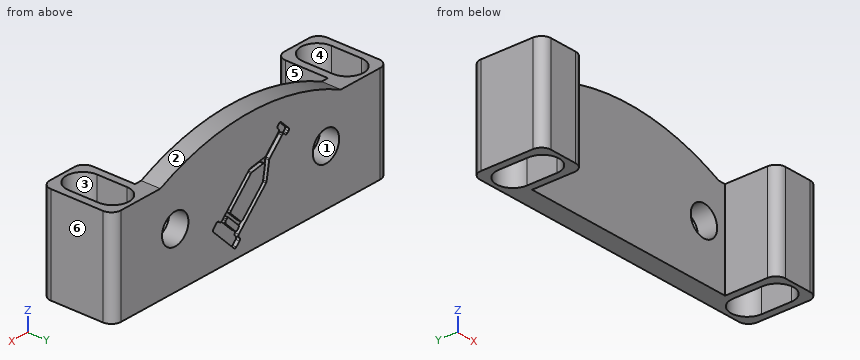
```python
from build123d import *

# Parameters (mm, degrees)
SKETCH_1_W          = 27.112781954
SKETCH_1_H          = 9.518796992
SKETCH_1_R          = 1.575
EXTRUDE_1_DEPTH     = 2
SKETCH_2_W          = 27.112781954
SKETCH_2_H          = 2
EXTRUDE_2_DEPTH     = 0.91
CUT_EXTRUDE_1_DEPTH = 15.829626281
CUT_EXTRUDE_2_DEPTH = 17.785702449
EXTRUDE_3_DEPTH     = 10
SKETCH_8_R          = 1.575
CUT_EXTRUDE_3_DEPTH = 10
EXTRUDE_4_DEPTH     = 2
FILLET_2_R          = 1
CUT_EXTRUDE_4_DEPTH = 0.4


with BuildPart() as part:
    # Эскиз1 → Бобышка-Вытянуть1 (new body)
    with BuildSketch(Plane(origin=(0, 0, 0), x_dir=(1, 0, 0), z_dir=(0, 1, 0))):
        Rectangle(SKETCH_1_W, SKETCH_1_H)
        with Locations(Location((-9, 0, 0), (0, 0, 270))):
            Circle(SKETCH_1_R, mode=Mode.SUBTRACT)
        with Locations(Location((9, 0, 0), (0, 0, 270))):
            Circle(SKETCH_1_R, mode=Mode.SUBTRACT)
    extrude(amount=EXTRUDE_1_DEPTH)

    # Эскиз2 → Бобышка-Вытянуть2 (add)
    with BuildSketch(Plane(origin=(0, 0, -4.759398496), x_dir=(-1, 0, 0), z_dir=(0, 0, -1))):
        with Locations((0, 1)):
            Rectangle(SKETCH_2_W, SKETCH_2_H)
    extrude(amount=EXTRUDE_2_DEPTH)

    # Эскиз3 → Вырез-Вытянуть1 (cut, through all)
    with BuildSketch(Plane.XZ):
        Polygon((-6.720997268, 4.759398496), (-3, 5.765), (-14.556442119, 5.765), (-14.556442119, -5.765), (-3, -5.765), (-3.353751395, -5.669398496), (-13.556390977, -5.669398496), (-13.556390977, 4.759398496), align=None)
        with BuildLine():
            Line((-10.043565082, 3.861472766), (-6.720997268, 4.759398496))
            Line((-6.720997268, 4.759398496), (-13.556390977, 4.759398496))
            Line((-13.556390977, 4.759398496), (-13.556390977, -5.669398496))
            Line((-13.556390977, -5.669398496), (-3.353751395, -5.669398496))
            Line((-3.353751395, -5.669398496), (-10.043565082, -3.861472766))
            ThreePointArc((-10.043565082, -3.861472766), (-13, 0), (-10.043565082, 3.861472766))
        make_face()
        with BuildLine():
            Line((13.556390977, 4.759398496), (6.720997268, 4.759398496))
            Line((6.720997268, 4.759398496), (10.043565082, 3.861472766))
            ThreePointArc((10.043565082, 3.861472766), (12.17602427, 2.431639331), (13, 0))
            ThreePointArc((13, 0), (12.17602427, -2.431639331), (10.043565082, -3.861472766))
            Line((10.043565082, -3.861472766), (3.353751395, -5.669398496))
            Line((3.353751395, -5.669398496), (13.556390977, -5.669398496))
            Line((13.556390977, -5.669398496), (13.556390977, 4.759398496))
        make_face()
        Polygon((3, 5.765), (6.720997268, 4.759398496), (13.556390977, 4.759398496), (13.556390977, -5.669398496), (3.353751395, -5.669398496), (3, -5.765), (14.556442119, -5.765), (14.556442119, 5.765), align=None)
    extrude(amount=-CUT_EXTRUDE_1_DEPTH, mode=Mode.SUBTRACT)

    # Эскиз4 → Вырез-Вытянуть2 (cut, through all)
    with BuildSketch(Plane(origin=(0, 0, -5.669398496), x_dir=(-1, 0, 0), z_dir=(0, 0, -1))):
        Polygon((11.521782541, 2), (11.521782541, -6.403006286), (13.618299284, -6.403006286), (13.618299284, 3.686124148), (11.521782541, 3.686124148), align=None)
        Polygon((-13.618299284, -6.403006286), (-11.521782541, -6.403006286), (-11.521782541, 2), (-11.521782541, 3.686124148), (-13.618299284, 3.686124148), align=None)
    extrude(amount=-CUT_EXTRUDE_2_DEPTH, mode=Mode.SUBTRACT)

    # Эскиз7 → Бобышка-Вытянуть3 (add)
    with BuildSketch(Plane(origin=(0, 0, -5.669398496), x_dir=(-1, 0, 0), z_dir=(0, 0, -1))):
        Polygon((3.353751395, 0), (11.521782541, 0), (11.521782541, -5.430586026), (16.478217459, -5.430586026), (16.478217459, 2), (11.521782541, 2), (3.353751395, 2), align=None)
        with BuildLine():
            Line((15.7, -3.265293013), (15.7, -0.165293013))
            ThreePointArc((15.7, -0.165293013), (14, 1.534706987), (12.3, -0.165293013))
            Line((12.3, -0.165293013), (12.3, -3.265293013))
            ThreePointArc((12.3, -3.265293013), (14, -4.965293013), (15.7, -3.265293013))
        make_face(mode=Mode.SUBTRACT)
    extrude_3 = extrude(amount=-EXTRUDE_3_DEPTH)

    # Эскиз8 → Вырез-Вытянуть3 (cut)
    with BuildSketch(Plane(origin=(0, 2, 0), x_dir=(1, 0, 0), z_dir=(0, 1, 0))):
        with Locations(Location((-9, 0, 0), (0, 0, 270))):
            Circle(SKETCH_8_R)
    cut_extrude_3 = extrude(amount=-CUT_EXTRUDE_3_DEPTH, mode=Mode.SUBTRACT)

    # Зеркальное отражение1: Бобышка-Вытянуть3, Вырез-Вытянуть3 across plane
    add(extrude_3.mirror(Plane(origin=(0, 0, 0), x_dir=(0, 0, 1), z_dir=(1, 0, 0))))
    add(cut_extrude_3.mirror(Plane(origin=(0, 0, 0), x_dir=(0, 0, 1), z_dir=(1, 0, 0))), mode=Mode.SUBTRACT)

    # Эскиз9 → Бобышка-Вытянуть4 (add)
    with BuildSketch(Plane(origin=(0, 2, 0), x_dir=(1, 0, 0), z_dir=(0, 1, 0))):
        with BuildLine():
            Line((6.720997268, -4.759398496), (-6.720997268, -4.759398496))
            Line((-6.720997268, -4.759398496), (-8.307661997, -4.330601504))
            Line((-8.307661997, -4.330601504), (-10.777839616, -4.330601504))
            ThreePointArc((-10.777839616, -4.330601504), (0, -6.773159867), (10.777839616, -4.330601504))
            Line((10.777839616, -4.330601504), (8.307661997, -4.330601504))
            Line((8.307661997, -4.330601504), (6.720997268, -4.759398496))
        make_face()
    extrude(amount=-EXTRUDE_4_DEPTH)

    # Скругление2
    fillet_2_edges = [part.edges().sort_by_distance(p)[0] for p in [
        (-16.478217459, 2, -0.669398496),
        (-16.478217459, -5.430586026, -0.669398496),
        (-11.521782541, -5.430586026, -0.669398496),
        (11.521782541, -5.430586026, -0.669398496),
        (16.478217459, -5.430586026, -0.669398496),
        (16.478217459, 2, -0.669398496),
    ]]
    fillet(fillet_2_edges, radius=FILLET_2_R)

    # Эскиз12 → Вырез-Вытянуть4 (cut)
    with BuildSketch(Plane(origin=(0, 2, 0), x_dir=(1, 0, 0), z_dir=(0, 1, 0))):
        with BuildLine():
            Line((4.446560813, 2.176089775), (1.988755362, 4.633895225))
            ThreePointArc((1.988755362, 4.633895225), (1.847334006, 4.692473869), (1.70591265, 4.633895225))
            Line((1.70591265, 4.633895225), (1.327376273, 4.255358849))
            ThreePointArc((1.327376273, 4.255358849), (1.268797629, 4.113937492), (1.327376273, 3.972516136))
            Line((1.327376273, 3.972516136), (1.402795262, 3.897097148))
            ThreePointArc((1.402795262, 3.897097148), (1.461373905, 3.755675791), (1.402795262, 3.614254435))
            Line((1.402795262, 3.614254435), (-1.852293326, 0.359165847))
            ThreePointArc((-1.852293326, 0.359165847), (-1.888439649, 0.309775569), (-1.907956953, 0.25176668))
            Line((-1.907956953, 0.25176668), (-2.218358166, -1.546336835))
            ThreePointArc((-2.218358166, -1.546336835), (-2.23787547, -1.604345724), (-2.274021793, -1.653736003))
            Line((-2.274021793, -1.653736003), (-3.75824321, -3.13795742))
            ThreePointArc((-3.75824321, -3.13795742), (-3.899664566, -3.196536063), (-4.041085922, -3.13795742))
            Line((-4.041085922, -3.13795742), (-4.109500023, -3.069543319))
            ThreePointArc((-4.109500023, -3.069543319), (-4.250921379, -3.010964675), (-4.392342735, -3.069543319))
            Line((-4.392342735, -3.069543319), (-4.522380617, -3.1995812))
            ThreePointArc((-4.522380617, -3.1995812), (-4.58095926, -3.341002556), (-4.522380617, -3.482423913))
            Line((-4.522380617, -3.482423913), (-3.669758325, -4.335046204))
            ThreePointArc((-3.669758325, -4.335046204), (-3.528336969, -4.393624848), (-3.386915613, -4.335046204))
            Line((-3.386915613, -4.335046204), (-3.256877732, -4.205008323))
            ThreePointArc((-3.256877732, -4.205008323), (-3.198299088, -4.063586966), (-3.256877732, -3.92216561))
            Line((-3.256877732, -3.92216561), (-3.325291832, -3.853751509))
            ThreePointArc((-3.325291832, -3.853751509), (-3.383870476, -3.712330153), (-3.325291832, -3.570908797))
            Line((-3.325291832, -3.570908797), (-1.841070415, -2.08668738))
            ThreePointArc((-1.841070415, -2.08668738), (-1.791680137, -2.050541057), (-1.733671248, -2.031023753))
            Line((-1.733671248, -2.031023753), (0.064432267, -1.720622541))
            ThreePointArc((0.064432267, -1.720622541), (0.122441156, -1.701105237), (0.171831435, -1.664958913))
            Line((0.171831435, -1.664958913), (3.426920022, 1.590129674))
            ThreePointArc((3.426920022, 1.590129674), (3.568341379, 1.648708318), (3.709762735, 1.590129674))
            Line((3.709762735, 1.590129674), (3.785181724, 1.514710686))
            ThreePointArc((3.785181724, 1.514710686), (3.92660308, 1.456132042), (4.068024436, 1.514710686))
            Line((4.068024436, 1.514710686), (4.446560813, 1.893247062))
            ThreePointArc((4.446560813, 1.893247062), (4.505139456, 2.034668419), (4.446560813, 2.176089775))
        make_face()
        with BuildLine():
            Line((2.963799211, 2.036003209), (1.848668796, 3.151133624))
            ThreePointArc((1.848668796, 3.151133624), (1.70724744, 3.209712267), (1.565826084, 3.151133624))
            Line((1.565826084, 3.151133624), (1.465360653, 3.050668193))
            ThreePointArc((1.465360653, 3.050668193), (1.406782009, 2.909246836), (1.465360653, 2.76782548))
            Line((1.465360653, 2.76782548), (2.580491067, 1.652695065))
            ThreePointArc((2.580491067, 1.652695065), (2.721912424, 1.594116422), (2.86333378, 1.652695065))
            Line((2.86333378, 1.652695065), (2.963799211, 1.753160497))
            ThreePointArc((2.963799211, 1.753160497), (3.022377855, 1.894581853), (2.963799211, 2.036003209))
        make_face(mode=Mode.SUBTRACT)
        with BuildLine():
            Line((2.334078689, 1.406282687), (1.218948275, 2.521413102))
            ThreePointArc((1.218948275, 2.521413102), (1.077526918, 2.579991746), (0.936105562, 2.521413102))
            Line((0.936105562, 2.521413102), (-1.42428076, 0.16102678))
            ThreePointArc((-1.42428076, 0.16102678), (-1.460427083, 0.111636501), (-1.479944387, 0.053627613))
            Line((-1.479944387, 0.053627613), (-1.712610446, -1.294168861))
            ThreePointArc((-1.712610446, -1.294168861), (-1.656946819, -1.469612406), (-1.481503274, -1.525276034))
            Line((-1.481503274, -1.525276034), (-0.1337068, -1.292609974))
            ThreePointArc((-0.1337068, -1.292609974), (-0.075697911, -1.27309267), (-0.026307633, -1.236946347))
            Line((-0.026307633, -1.236946347), (2.334078689, 1.123439975))
            ThreePointArc((2.334078689, 1.123439975), (2.392657333, 1.264861331), (2.334078689, 1.406282687))
        make_face(mode=Mode.SUBTRACT)
    extrude(amount=-CUT_EXTRUDE_4_DEPTH, mode=Mode.SUBTRACT)


solid = part.part
```
The listing builds one solid part. Answer for the finished solid, in the listing's coordinates (mm). Face numbers are marked on the shaded views. A direction names the side the tool comes from. Give positions to 0.01 mm unless a question says otherwise; leave off trailing zeros. Write each loop counter-clockwise with the first axis right and the second up, starting at its lowest first coordinate (ties: lowest second). Pieces come first, ordered by that corner, then holes. Notation, with made-up numbers: M 23,-17.75 L 53,-17.75 A31 cw 53,9.25 Z; hole C -23.5,33.25 d11. An arc over 180 degrees is marked long. Write each question's results on one line, items separated by ' | '.
Q1. Section A-A, the plane x = -14 is taken. Write down the section's boundary in (y, z).
Output values:
outline: M -5.43,-5.67 L -4.97,-5.67 L -4.97,4.33 L -5.43,4.33 Z; M 1.53,-5.67 L 2,-5.67 L 2,4.33 L 1.53,4.33 Z
Q2. Flat-ended cylindrical pins translate along their axes: P1, Ø3, axis at x = -5.5, z = -3, coming from the -Y side; P2, Ø3, axis at x = 9, z = 0, coming from the -Y side. Find the tip coordinate at first contact, or state that the pin passes through.
Output values:
P1: y = 0 | P2: through
Q3. A tool of negligible diameter and unlimited length cuts with its end or side. For the marked faces 4, 5 and 6, from which of +Z, -Z, +X, -X, +Y, -Y can it reach the whole face along a straight path? Write none if from no direction.
Output values:
face 4: +Z, -Z | face 5: +Z, -Z, -Y | face 6: +Z, -Z, +X, +Y, -Y
Q4. Consider L1, parallel to X at y = -1.5, z = 0.5; L2, parallel to X at y = -4.25, z = 2.5; L3, parallel to Y at x = 14, z = 4.25. Determine where each line is inside the solid, lowest interval first. Write a range as from..to.
Output values:
L1: -16.48..-15.7, -12.3..-11.52, 11.52..12.3, 15.7..16.48 | L2: -16.48..-15.39, -12.61..-11.52, 11.52..12.61, 15.39..16.48 | L3: -5.43..-4.97, 1.53..2
Q5. Section C-C, the plane x = 9 is taken. Write down the section's boundary in (y, z) (3 decimals).
Output values:
outline: M 0,-5.669 L 2,-5.669 L 2,-1.575 L 0,-1.575 Z; M 0,1.575 L 2,1.575 L 2,5.097 L 0,5.097 Z
Q6. For a pull along Z with two mould halves and no side action, classify the marked faces 1, 2 and 3 as released by +Z, released by -Z, zero draft, split by the parting line, or undercut.
Output values:
face 1: undercut | face 2: released by +Z | face 3: zero draft
Q7. Section D-D, the plane z = 5 is taken. Write down the section's boundary in (x, y), then the cut area to 3 significant figures.
Output values:
outline: M -9.25,0 L 9.25,0 L 9.25,2 L -9.25,2 Z | area: 37.0 mm2
Q8. Section B-B, the plane y = -0.75 is taken. Write down the section's boundary in (x, z).
Output values:
outline: M -16.48,-5.67 L -15.7,-5.67 L -15.7,4.33 L -16.48,4.33 Z; M -12.3,-5.67 L -11.52,-5.67 L -11.52,4.33 L -12.3,4.33 Z; M 11.52,-5.67 L 12.3,-5.67 L 12.3,4.33 L 11.52,4.33 Z; M 15.7,-5.67 L 16.48,-5.67 L 16.48,4.33 L 15.7,4.33 Z
